from build123d import *

# Parameters (mm, degrees)
SKETCH_1_R      = 1.5
SKETCH_1_W      = 10
SKETCH_1_H      = 4
SKETCH_1_R_2    = 10
SKETCH_1_R_3    = 4.5
EXTRUDE_1_DEPTH = 3
FILLET_1_R      = 3.8


with BuildPart() as part:
    # 草图1 → 凸台-拉伸1 (new body)
    with BuildSketch(Plane(origin=(0, 0, 0), x_dir=(1, 0, 0), z_dir=(0, 1, 0))):
        Polygon((195.7, 16), (195.7, 0), (203.2, 0), (203.2, 50.673), (0, 50.673), (0, 0), (8.129, 0), (11.129, 6), (21.129, 6), (24.129, 0), (35, 0), (35, 10), (61.620357325, 10), (79.620357325, 10), (81, 10), (92, 10), (95, 0), (110.764, 0), (110.764, 9), (116.764, 9), (116.764, 19), (143.764, 19), (143.764, 0), (169.7, 0), (169.7, 8), (186.7, 8), (186.7, 16), align=None)
        with Locations((4.064, 4.064)):
            Circle(SKETCH_1_R, mode=Mode.SUBTRACT)
        with Locations((31.242, 19.05)):
            Rectangle(SKETCH_1_W, SKETCH_1_H, mode=Mode.SUBTRACT)
        with Locations((199.39, 4.064)):
            Circle(SKETCH_1_R, mode=Mode.SUBTRACT)
        with Locations((21.336, 35.673)):
            Circle(SKETCH_1_R_2, mode=Mode.SUBTRACT)
        with Locations((48.641, 35.673)):
            Circle(SKETCH_1_R_2, mode=Mode.SUBTRACT)
        with Locations((68.691, 35.306)):
            Circle(SKETCH_1_R_3, mode=Mode.SUBTRACT)
        with Locations((87.884, 35.673)):
            Circle(SKETCH_1_R_2, mode=Mode.SUBTRACT)
        with Locations((4.318, 47.371)):
            Circle(SKETCH_1_R, mode=Mode.SUBTRACT)
        with Locations((115.316, 35.673)):
            Circle(SKETCH_1_R_2, mode=Mode.SUBTRACT)
        with Locations((134.493, 35.306)):
            Circle(SKETCH_1_R_3, mode=Mode.SUBTRACT)
        with Locations((154.432, 35.673)):
            Circle(SKETCH_1_R_2, mode=Mode.SUBTRACT)
        with Locations((181.737, 35.673)):
            Circle(SKETCH_1_R_2, mode=Mode.SUBTRACT)
        with Locations((199.39, 47.498)):
            Circle(SKETCH_1_R, mode=Mode.SUBTRACT)
    extrude(amount=EXTRUDE_1_DEPTH)

    # 圆角1
    fillet_1_edges = [part.edges().sort_by_distance(p)[0] for p in [
        (0, 1.5, 0),
        (0, 1.5, -50.673),
        (203.2, 1.5, -50.673),
        (203.2, 1.5, 0),
    ]]
    fillet(fillet_1_edges, radius=FILLET_1_R)


solid = part.part
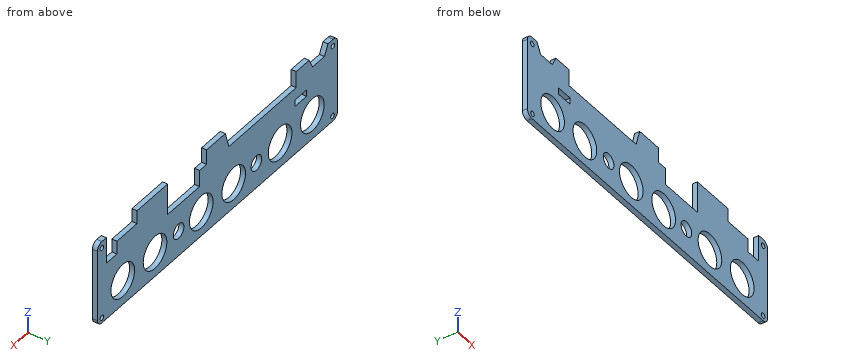
Read the model definition and answer for the solid it produces. Units are mm, in the model's axes. Coordinates: 2 decimals unless noted, no trailing zeros. Write each loop counter-clockwise with the first axis right and the second up, starting at its lowest first coordinate (ties: lowest second). Pieces come first, ordered by that corner, then holes. Notation, with made-up numbers: (39.5, 6.25) - (48.5, 6.25) arc R11 cw to (48.5, 26.25) - close; hole circle Ø9 at (60, -23). An arc over 180 degrees is marked (long way). One line per question, with ' | ' between items.
Q1. Find section B-B, the plane y = 2.3. State how many separate pieces and enclosed holes the cut face has, plus the area to 3 significant figures.
Result set:
separate pieces: 1 | enclosed holes: 13 | area: 6,690 mm^2
Q2. Find section A-A, the plane x = 107.5. Write down the section's boundary in (y, z).
Result set:
outline: (0, -50.67) - (3, -50.67) - (3, -41.91) - (0, -41.91) - close; (0, -29.44) - (3, -29.44) - (3, 0) - (0, 0) - close
Q3. Consider L1, parallel to X at y = 2.15, z = -10.5; L2, parallel to X at y = 0.2, z = -1.5; L3, parallel to X at y = 0.85, z = -48. Determine where each line is inside the solid, lowest interval first. Write a range as [from, to].
Result set:
L1: [0, 116.76], [143.76, 186.7], [195.7, 203.2] | L2: [0.78, 8.88], [23.38, 35], [94.55, 110.76], [143.76, 169.7], [195.7, 202.42] | L3: [0.17, 2.96], [5.68, 197.98], [200.8, 203.03]
